For this review, take the finished solid that the model builds, in its own axes (mm). A direction names the side the tool comes from. Coordinates: 2 decimals unless noted, no trailing zeros. Order: outer loops, then holes, each group sorted by start corner. A loop starts at its lowest first (then second) coordinate and runs counter-clockwise, first axis right, second up. Notation, with made-up numbers: (1.25, -3.5) -> (20.25, -3.5) arc R26 cw to (20.25, 28.5) -> close; hole circle Ø6 at (15.5, 80.25). An arc over 180 degrees is marked (long way). Write item = value, one per line. Start each with the question number.
1) Consider section D-D on x = 19.5. Give the boundary of the cut face in (y, z), and give its area (3 significant figures).
2) Consider section B-B on y = -8. Give the boundary of the cut face in (x, z).
3) Draft analysis for pull direction X (two halves, no side actions). For faces 3 (the face through (-41.515, -31, -18)), 4 (the face through (34.685, -15, -7)), 5 (the face through (47.21, -17.76, 2.38)), state which applies: +X half, -X half, draft (parallel to the pull), parting line (faces both ways), or undercut.
4) Wall thickness on probe 1 along X at (y, z) = (-3.5, -12); probe 2 along Y at (x, z) = (16.5, 1); probe 3 along Z at (x, y) = (6, -6): over which ranges is each line inside the solid? List them lowest first. Write a range as [from, to].
5) Insertion check: pin 1 Ø11.5 at (x, z) = (-1.5, -4.5) entering from +Y; pin 2 Ø7.5 at (x, y) = (18.5, -8.5) entering from +Z; pin 3 Ø10 at (x, z) = (43.5, 6) entering from +Y. Each pin has a flat end and moves straight along its axis. Give the tip position at first contact, or say it passes through.
6) Consider section A-A on x = 49. Give the boundary of the cut face in (y, z), and give its area (3 significant figures).
7) Machinability: for faces 1 (the face through (60.085, -31, -18)), 2 (the face through (10, -13, -17.561)), which of the approach directions +Z, -Z, +X, -X, +Y, -Y give a long, thin tool a straight path to every point of the face, cutting with its end or side? Answer none if there is none.
8) Consider section C-C on y = -20.5. Give the boundary of the cut face in (x, z).
from build123d import *

# Parameters (mm, degrees)
F0_W     = 101.6
F0_H     = 76.2
F1_DEPTH = 63.5
F2_W     = 50.8
F2_H     = 38.1
F3_DEPTH = 25.4
F5_DEPTH = 101.601


with BuildPart() as f1:
    # F0 (on Front) → F1 (new body)
    with BuildSketch(Plane.XZ):
        with Locations((9.285491, -17.560551)):
            Rectangle(F0_W, F0_H)
    extrude(amount=F1_DEPTH)

    # F2 (on face) → F3 (cut)
    with BuildSketch(Plane(origin=(0, 0, 0), x_dir=(-1, 0, 0), z_dir=(0, 1, 0))):
        with Locations((-9.285491, 1.489449)):
            Rectangle(F2_W, F2_H)
    extrude(amount=-F3_DEPTH, mode=Mode.SUBTRACT)

    # F4 (on face) → F5 (cut, through all)
    with BuildSketch(Plane(origin=(-41.514509, 0, 0), x_dir=(0, -1, 0), z_dir=(-1, 0, 0))):
        with BuildLine():
            Line((0, 20.539449), (0, -4.860551))
            ThreePointArc((0, -4.860551), (17.960512, 2.578937), (25.4, 20.539449))
            Line((25.4, 20.539449), (0, 20.539449))
        make_face()
    extrude(amount=-F5_DEPTH, mode=Mode.SUBTRACT)


solid = f1.part
Answer sheet:
q1.outline = (-63.5, -55.66) -> (0, -55.66) -> (0, -17.56) -> (-25.4, -17.56) -> (-25.4, 20.54) -> (-63.5, 20.54) -> close
q1.area = 3,870 mm2
q2.outline = (-41.51, -55.66) -> (60.09, -55.66) -> (60.09, -3.57) -> (34.69, -3.57) -> (34.69, -17.56) -> (-16.11, -17.56) -> (-16.11, -3.57) -> (-41.51, -3.57) -> close
q3.face_3 = -X half
q3.face_4 = undercut
q3.face_5 = draft
q4.probe_1 = [-41.51, -16.11], [34.69, 60.09]
q4.probe_2 = [-63.5, -25.4]
q4.probe_3 = [-55.66, -17.56]
q5.pin_1 = -25.4
q5.pin_2 = -17.56
q5.pin_3 = -16.23
q6.outline = (-63.5, -55.66) -> (0, -55.66) -> (0, -4.86) arc R25.4 cw to (-25.4, 20.54) -> (-63.5, 20.54) -> close
q6.area = 4,330 mm2
q7.face_1 = +Z, -Z, +X, +Y, -Y
q7.face_2 = +Z, +Y
q8.outline = (-41.51, -55.66) -> (60.09, -55.66) -> (60.09, 5.54) -> (34.69, 5.54) -> (34.69, -17.56) -> (-16.11, -17.56) -> (-16.11, 5.54) -> (-41.51, 5.54) -> close
